Work out the finished part from the listing and answer in its coordinate system (mm). Face numbers are marked on the shaded views. A direction names the side the tool comes from. Give positions to 0.01 mm unless a question says otherwise; leave off trailing zeros. Loops run counter-clockwise (first coordinate to the right, second up) from the corner with the lowest first, then second, coordinate; pieces in that order, holes last. Notation, with made-up numbers: (62, 21) - (87, 21) arc R33 cw to (87, 58) - close; hole circle Ø7 at (78, 55). An arc over 180 degrees is marked (long way). One line per item, written item: value.
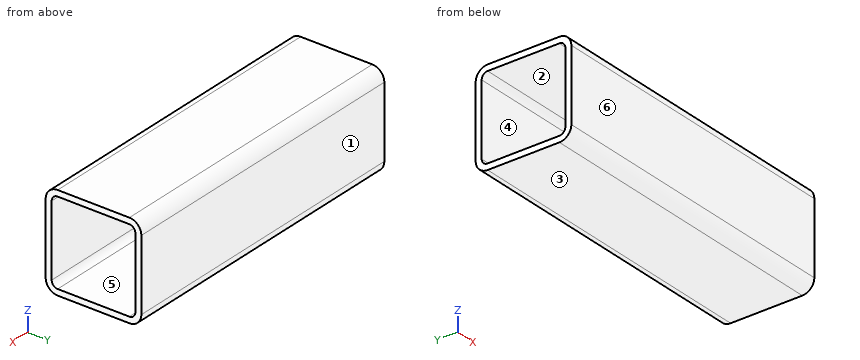
from build123d import *

# Parameters (mm, degrees)
F1_DEPTH = 130


with BuildPart() as f1:
    # F0 (on Right) → F1 (new body, symmetric)
    with BuildSketch(Plane.YZ):
        with BuildLine():
            ThreePointArc((40, 30), (37.071068, 37.071068), (30, 40))
            Line((30, 40), (-30, 40))
            ThreePointArc((-30, 40), (-37.071068, 37.071068), (-40, 30))
            Line((-40, 30), (-40, -30))
            ThreePointArc((-40, -30), (-37.071068, -37.071068), (-30, -40))
            Line((-30, -40), (30, -40))
            ThreePointArc((30, -40), (37.071068, -37.071068), (40, -30))
            Line((40, -30), (40, 30))
        make_face()
        with BuildLine():
            ThreePointArc((30, 35), (33.535534, 33.535534), (35, 30))
            Line((35, 30), (35, -30))
            ThreePointArc((35, -30), (33.535534, -33.535534), (30, -35))
            Line((30, -35), (-30, -35))
            ThreePointArc((-30, -35), (-33.535534, -33.535534), (-35, -30))
            Line((-35, -30), (-35, 30))
            ThreePointArc((-35, 30), (-33.535534, 33.535534), (-30, 35))
            Line((-30, 35), (30, 35))
        make_face(mode=Mode.SUBTRACT)
    extrude(amount=F1_DEPTH, both=True)


solid = f1.part
1. For the marked faces 5 and 6, determine the directions among +Z, -Z, +X, -X, +Y, -Y from which every point of the face is accessible in a straight line to the end or side of a thin tool.
Output:
face 5: +X, -X
face 6: +Z, -Z, +X, -X, -Y
2. Find the intervals of material crossed by line 1 along Y through (x, z) = (-108, -7.5); line 2 along Z through (x, y) = (20.5, -33.5), in increasing order.
Output:
line 1: y = -40 to -35, 35 to 40
line 2: z = -39.37 to -33.57, 33.57 to 39.37
3. Section A-A (y = -16) is taken. Write down the section's boundary in (x, z).
Output:
outline: (-130, -40) - (130, -40) - (130, -35) - (-130, -35) - close; (-130, 35) - (130, 35) - (130, 40) - (-130, 40) - close
4. The mould has two halves that part along Y. Classify the marked faces 1, 2, 3 and 4: released by +Y, released by -Y, zero draft, split by the parting line, or undercut.
Output:
face 1: released by +Y
face 2: undercut
face 3: zero draft
face 4: undercut
5. Section C-C (x = 99) is taken. Write down the section's boundary in (y, z).
Output:
outline: (-40, -30) arc R10 ccw to (-30, -40) - (30, -40) arc R10 ccw to (40, -30) - (40, 30) arc R10 ccw to (30, 40) - (-30, 40) arc R10 ccw to (-40, 30) - close; hole (-35, -30) arc R5 ccw to (-30, -35) - (30, -35) arc R5 ccw to (35, -30) - (35, 30) arc R5 ccw to (30, 35) - (-30, 35) arc R5 ccw to (-35, 30) - close
